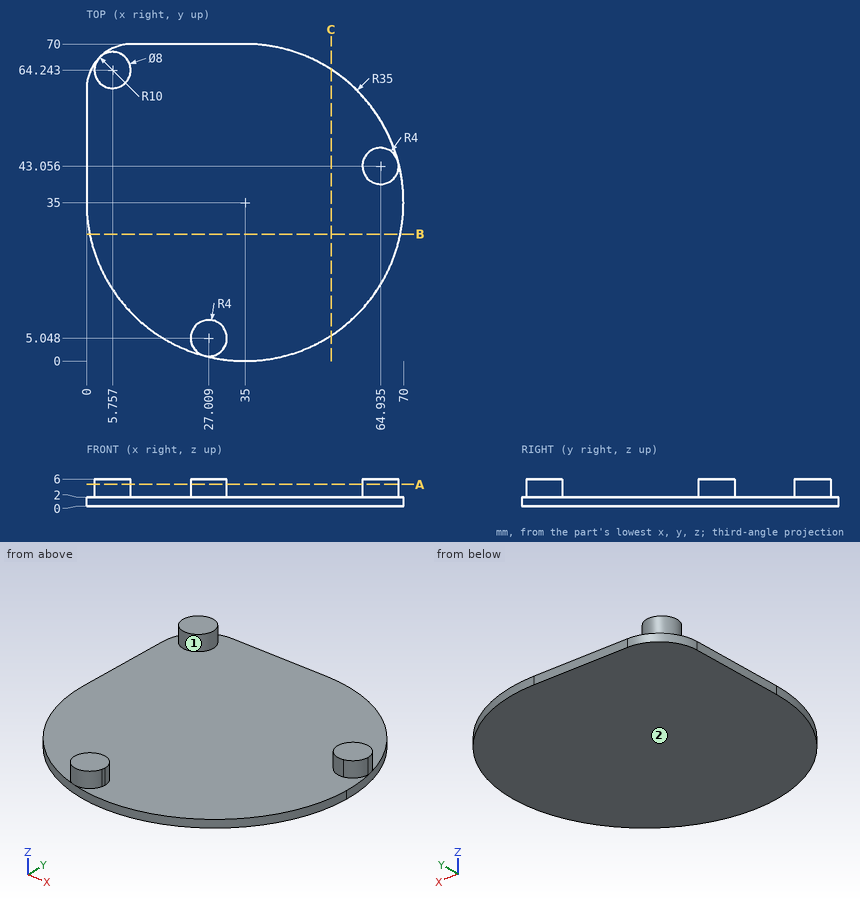
Drawing for the job (mm, zero at the part's lowest x, y, z). A direction names the side the tool comes from. Round coordinates to 2 decimals unless told otherwise and drop trailing zeros. Write each loop counter-clockwise with the first axis right and the second up, starting at its lowest first coordinate (ties: lowest second). Pieces come first, ordered by that corner, then holes.
Item 1: Band-saw the part on B-B on y = 28. Write the cut outline in (x, z).
Filled in:
outline: (0.71, 0) - (69.29, 0) - (69.29, 2) - (0.71, 2) - close
Item 2: Drop flat-ended pins along their axis: pin 1 Ø2 at (x, y) = (60, 57) entering from +Z; pin 2 Ø1.5 at (y, z) = (22.5, 2) entering from +X. Give the stop position or say it passes through.
Filled in:
pin 1: stops at z = 2
pin 2: stops at x = 67.97
Item 3: Band-saw the part on C-C on x = 54. Write the cut outline in (y, z).
Filled in:
outline: (5.61, 0) - (64.39, 0) - (64.39, 2) - (5.61, 2) - close
Item 4: Drill centre lines: L1, parallel to Z at x = 22.5, y = 11; L2, parallel to X at y = 46, z = 0.65; L3, parallel to X at y = 44.5, z = 1.25 (1 decimal). Where is each one in solid material? Low to high.
Filled in:
L1: z = 0 to 2
L2: x = 0 to 68.23
L3: x = 0 to 68.7
Item 5: Tool access for the marked faces 1 and 2: list every direction of +Z, -Z, +X, -X, +Y, -Y with a clear straight run to the whole face (end or side of a thin tool).
Filled in:
face 1: +Z
face 2: -Z, +X, -X, +Y, -Y
Item 6: Band-saw the part on A-A on z = 4.8. Write the cut outline in (x, y) (1 decimal), then the cut area to 3 significant figures.
Filled in:
outline: circle Ø8 at (5.8, 64.2); circle Ø8 at (27, 5); circle Ø8 at (64.9, 43.1)
area: 151 mm2
